from build123d import *

# Parameters (mm, degrees)
SKETCH1_R               = 70
BOSS_EXTRUDE1_DEPTH     = 7.5
FILLET1_R               = 3
CUT_EXTRUDE2_DEPTH      = 100.278648258
CUT_EXTRUDE2_DEPTH_BACK = 100.278648258
CUT_EXTRUDE3_DEPTH      = 98.628141683
CUT_EXTRUDE3_DEPTH_BACK = 98.628141683
FILLET2_R               = 14
FILLET3_R               = 3


with BuildPart() as part:
    # Sketch1 → Boss-Extrude1 (new, symmetric)
    with BuildSketch(Plane.XY):
        Circle(SKETCH1_R)
        Polygon((23.094010768, 0), (11.547005384, 20), (-11.547005384, 20), (-23.094010768, 0), (-11.547005384, -20), (11.547005384, -20), align=None, mode=Mode.SUBTRACT)
    extrude(amount=BOSS_EXTRUDE1_DEPTH, both=True)

    # Fillet1
    fillet1_edges = [part.edges().sort_by_distance(p)[0] for p in [
        (23.094010768, 0, 0),
        (11.547005384, 20, 0),
        (-11.547005384, 20, 0),
        (-23.094010768, 0, 0),
        (-11.547005384, -20, 0),
        (11.547005384, -20, 0),
    ]]
    fillet(fillet1_edges, radius=FILLET1_R)

    # Sketch3 → Cut-Extrude2 (cut, two sides)
    with BuildSketch(Plane.XY) as cut_extrude2_sk:
        with BuildLine():
            ThreePointArc((63.398675482, 29.675039126), (40.067343971, 57.398675482), (6, 69.742383097))
            Line((6, 69.742383097), (12, 68.467043727))
            Line((12, 68.467043727), (5.525264217, 61.276121136))
            ThreePointArc((5.525264217, 61.276121136), (36.300148732, 55.601545074), (59.006370637, 34.067343971))
            Line((59.006370637, 34.067343971), (63.398675482, 29.675039126))
        make_face()
        with BuildLine():
            ThreePointArc((-50.304045441, 35.423079743), (-30.002276158, 59.2376235), (0, 68.134687942))
            Line((0, 68.134687942), (0, 70))
            ThreePointArc((0, 70), (-32.367313157, 62.067358885), (-57.398675482, 40.067343971))
            Line((-57.398675482, 40.067343971), (-53.294199189, 44.625826709))
            Line((-53.294199189, 44.625826709), (-50.304045441, 35.423079743))
        make_face()
        with BuildLine():
            ThreePointArc((70, 0), (68.329742001, 15.200209147), (63.398675482, 29.675039126))
            Line((63.398675482, 29.675039126), (65.294199189, 23.841217018))
            Line((65.294199189, 23.841217018), (55.829309658, 25.853041393))
            ThreePointArc((55.829309658, 25.853041393), (66.30242489, -3.636078426), (59.006370637, -34.067343971))
            Line((59.006370637, -34.067343971), (57.398675482, -40.067343971))
            ThreePointArc((57.398675482, -40.067343971), (66.77539698, -21.001103736), (70, 0))
        make_face()
        with BuildLine():
            Line((-59.006370637, 34.067343971), (-57.398675482, 40.067343971))
            ThreePointArc((-57.398675482, 40.067343971), (-69.742383097, 6), (-63.398675482, -29.675039126))
            Line((-63.398675482, -29.675039126), (-65.294199189, -23.841217018))
            Line((-65.294199189, -23.841217018), (-55.829309658, -25.853041393))
            ThreePointArc((-55.829309658, -25.853041393), (-66.30242489, 3.636078426), (-59.006370637, 34.067343971))
        make_face()
        with BuildLine():
            Line((-59.006370637, -34.067343971), (-63.398675482, -29.675039126))
            ThreePointArc((-63.398675482, -29.675039126), (-40.067343971, -57.398675482), (-6, -69.742383097))
            Line((-6, -69.742383097), (-12, -68.467043727))
            Line((-12, -68.467043727), (-5.525264217, -61.276121136))
            ThreePointArc((-5.525264217, -61.276121136), (-36.300148732, -55.601545074), (-59.006370637, -34.067343971))
        make_face()
        with BuildLine():
            Line((0, -68.134687942), (-6, -69.742383097))
            ThreePointArc((-6, -69.742383097), (29.675039126, -63.398675482), (57.398675482, -40.067343971))
            Line((57.398675482, -40.067343971), (53.294199189, -44.625826709))
            Line((53.294199189, -44.625826709), (50.304045441, -35.423079743))
            ThreePointArc((50.304045441, -35.423079743), (30.002276158, -59.2376235), (0, -68.134687942))
        make_face()
    extrude(amount=CUT_EXTRUDE2_DEPTH, mode=Mode.SUBTRACT)
    extrude(cut_extrude2_sk.sketch, amount=-CUT_EXTRUDE2_DEPTH_BACK, mode=Mode.SUBTRACT)

    # Sketch4 → Cut-Extrude3 (cut, two sides)
    with BuildSketch(Plane.XY.offset(7.5)) as cut_extrude3_sk:
        Polygon((0, 68.134687942), (6, 69.742383097), (0, 70), align=None)
    extrude(amount=CUT_EXTRUDE3_DEPTH, mode=Mode.SUBTRACT)
    extrude(cut_extrude3_sk.sketch, amount=-CUT_EXTRUDE3_DEPTH_BACK, mode=Mode.SUBTRACT)


with BuildPart() as body_2:
    # of the pieces the cut leaves, the one that is kept (cut_extrude3_keep)
    add(part.part.solids().sort_by_distance((55.829309658, 25.853041393, 7.5))[0])

    # Fillet2
    fillet2_edges = [body_2.edges().sort_by_distance(p)[0] for p in [
        (63.398675482, 29.675039126, 0),
        (-57.398675482, 40.067343971, 0),
        (-59.006370637, -34.067343971, 0),
        (-6, -69.742383097, 0),
        (0, 68.134687942, 0),
        (0, -68.134687942, 0),
        (57.398675482, -40.067343971, 0),
        (-59.006370637, 34.067343971, 0),
        (-63.398675482, -29.675039126, 0),
        (59.006370637, 34.067343971, 0),
        (6, 69.742383097, 0),
        (59.006370637, -34.067343971, 0),
    ]]
    fillet(fillet2_edges, radius=FILLET2_R)

    # Fillet3
    fillet3_edges = [body_2.edges().sort_by_distance(p)[0] for p in [
        (-50.304045441, 35.423079743, 0),
        (-5.525264217, -61.276121136, 0),
        (50.304045441, -35.423079743, 0),
        (-55.829309658, -25.853041393, 0),
        (5.525264217, 61.276121136, 0),
        (55.829309658, 25.853041393, 0),
    ]]
    fillet(fillet3_edges, radius=FILLET3_R)


solid = body_2.part
The listing builds one solid part. Answer for the finished solid, in the listing's coordinates (mm). A direction names the side the tool comes from. Give positions to 0.01 mm unless a question says otherwise; leave off trailing zeros. Write each loop counter-clockwise with the first axis right and the second up, starting at its lowest first coordinate (ties: lowest second). Pieces come first, ordered by that corner, then holes. Notation, with made-up numbers: (43.25, -11.75) - (100.25, -11.75) arc R9 ccw to (100.25, -5.75) - close; hole circle Ø4 at (-1, 67). An arc over 180 degrees is marked (long way). Use a Markdown table: item, result.
1. Section D-D on y = -50.5 is taken. Write down the section's boundary in (x, z), plus the area to 3 significant figures.
Values follow:
| item | result |
|---|---|
| outline | (-44.47, -7.5) - (40.37, -7.5) - (40.37, 7.5) - (-44.47, 7.5) - close |
| area | 1,270 mm² |
2. Section A-A on y = 14.5 is taken. Write down the section's boundary in (x, z), plus the area to 3 significant figures.
Values follow:
| item | result |
|---|---|
| outline | (-65.8, -7.5) - (-14.72, -7.5) - (-14.72, 7.5) - (-65.8, 7.5) - close; (14.72, -7.5) - (62.19, -7.5) - (62.19, 7.5) - (14.72, 7.5) - close |
| area | 1,480 mm² |
3. Find the intervals of material crossed by probe 1 along Y at (x, z) = (-10, 1); probe 2 along Y at (x, z) = (0.5, 6); probe 3 along Y at (x, z) = (-60.5, -2), in increasing order. Write a range as from..to.
Values follow:
| item | result |
|---|---|
| probe 1 | y = -68.89..-66.18, -62.96..-19.99, 19.99..67.22 |
| probe 2 | y = -68.18..-20, 20..68.32 |
| probe 3 | y = -32.57..-23.92, -18.2..31.3 |
4. Section C-C on x = 33.5 is taken. Write down the section's boundary in (y, z).
Values follow:
| item | result |
|---|---|
| outline | (-56.76, -7.5) - (56.93, -7.5) - (56.93, 7.5) - (-56.76, 7.5) - close |
5. For a pull along Y with two mould halves and no side action, classify faces 3 (the cylindrical face through (5.964, 69.343, -0.105)), 4 (the cylindrical face through (50.048, -40.164, -0.105)), 5 (the flat face through (-17.39, -9.88, 0.11)) as released by +Y, released by -Y, zero draft, split by the parting line, or undercut.
Values follow:
| item | result |
|---|---|
| face 3 | released by +Y |
| face 4 | released by -Y |
| face 5 | undercut |
6. A tool of negligible diameter and unlimited length cuts with its end or side. For faces 1 (the flat face through (17.39, 9.88, 0.11)), 2 (the cylindrical face through (57.07, -39.84, -0.11)), from which of +Z, -Z, +X, -X, +Y, -Y can it reach the whole face along a straight path? Write none if from no direction.
Values follow:
| item | result |
|---|---|
| face 1 | +Z, -Z |
| face 2 | +Z, -Z, +X, -Y |
7. Section B-B on x = -17 is taken. Write down the section's boundary in (y, z), plus the area to 3 significant figures.
Values follow:
| item | result |
|---|---|
| outline | (-61.29, -7.5) - (-10.56, -7.5) - (-10.56, 7.5) - (-61.29, 7.5) - close; (10.56, -7.5) - (65.44, -7.5) - (65.44, 7.5) - (10.56, 7.5) - close |
| area | 1,580 mm² |
8. Each of these flat-tipped pins is pushed along its axis until it touches: P1, Ø1.5, axis at x = 10, z = 0, coming from the +Y side; P2, Ø1.5, axis at x = 51.5, z = -4, coming from the +Y side; P3, Ø3, axis at x = 4, z = -5, coming from the +Y side. Where does it stop, or does it pass through?
Values follow:
| item | result |
|---|---|
| P1 | stops at y = 69.05 |
| P2 | stops at y = 44.97 |
| P3 | stops at y = 69.32 |
